Geometry check sheet. Reference: the model listing, model coordinates, mm. Face numbers are marked on the shaded views. A direction names the side the tool comes from. Round coordinates to 2 decimals unless told otherwise and drop trailing zeros. Write each loop counter-clockwise with the first axis right and the second up, starting at its lowest first coordinate (ties: lowest second). Pieces come first, ordered by that corner, then holes. Notation, with made-up numbers: M 86.5,-38.75 L 96.5,-38.75 A14 ccw 96.5,-14.75 Z; hole C 67.5,80.5 d7. An arc over 180 degrees is marked long. Use a Markdown table: item, result.
```python
from build123d import *

# Parameters (mm, degrees)
F1_DEPTH      = 12.7
F1_DEPTH_BACK = 12.7
F2_R          = 3.937
F3_DEPTH      = 25.401
F5_W          = 25.4239097328
F5_H          = 19.05
F6_DEPTH      = 20.9247035883
F6_DEPTH_BACK = 20.2536193136


with BuildPart() as f1:
    # F0 (on Front) → F1 (new body, two sides)
    with BuildSketch(Plane.XZ) as f1_sk:
        with BuildLine():
            Line((622.2402070197, 68.0433236969), (599.7125589726, 54.4963749958))
            ThreePointArc((599.7125589726, 54.4963749958), (596.4317742001, 46.7743526151), (602.7544880205, 41.259239895))
            Line((602.7544880205, 41.259239895), (604.0336175771, 41.259239895))
            Line((604.0336175771, 41.259239895), (628.785084933, 41.259239895))
            Line((628.785084933, 41.259239895), (644.685484933, 41.259239895))
            Line((644.685484933, 41.259239895), (644.685484933, 57.159639895))
            Line((644.685484933, 57.159639895), (641.485084933, 57.159639895))
            ThreePointArc((641.485084933, 57.159639895), (622.5332831727, 46.1050040009), (622.2402070197, 68.0433236969))
        make_face()
        with BuildLine():
            Line((604.0336175771, 41.259239895), (602.7544880205, 41.259239895))
            ThreePointArc((602.7544880205, 41.259239895), (603.3940527988, 41.2305528572), (604.0336175771, 41.259239895))
        make_face()
    extrude(amount=F1_DEPTH)
    extrude(f1_sk.sketch, amount=-F1_DEPTH_BACK)

    # F2 (on face) → F3 (cut, through all)
    with BuildSketch(Plane(origin=(0, 12.7, 0), x_dir=(-1, 0, 0), z_dir=(0, 1, 0))):
        with Locations((-603.3940527988, 48.3743028572)):
            Circle(F2_R)
    extrude(amount=-F3_DEPTH, mode=Mode.SUBTRACT)

    # F5 (on face) → F6 (cut, two sides)
    with BuildSketch(Plane(origin=(49.5651934259, 0, -143.2513532049), x_dir=(0.9450305474, 0, 0.3269820552), z_dir=(0.3269820552, 0, -0.9450305474))) as f6_sk:
        with Locations((584.3355135098, 0)):
            Rectangle(F5_W, F5_H)
    extrude(amount=-F6_DEPTH, mode=Mode.SUBTRACT)
    extrude(f6_sk.sketch, amount=F6_DEPTH_BACK, mode=Mode.SUBTRACT)


solid = f1.part
```
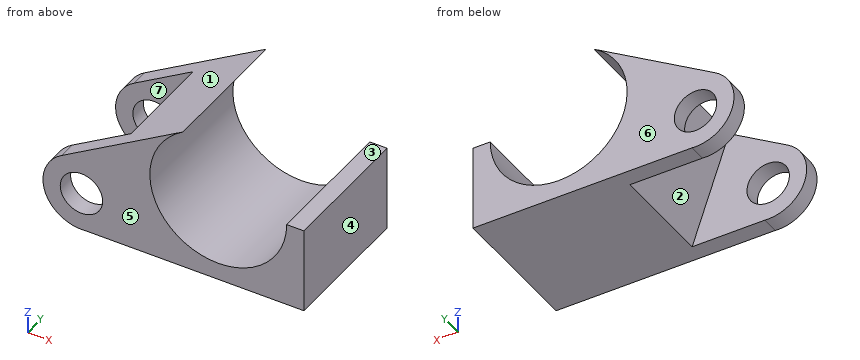
Item 1: Material ranges on line 1 along Y through (x, z) = (608.5, 57) (3 decimals); line 2 along X through (y, z) = (3, 56.25); line 3 along X through (y, z) = (7, 55.75), recorded low to high. Write a range as from..to.
Outcome:
| item | result |
|---|---|
| line 1 | y = -12.7..-9.525, 9.525..12.7 |
| line 2 | x = 612.31..616.12, 641.45..644.69 |
| line 3 | x = 612.49..616.16, 641.41..644.69 |
Item 2: Cross-section at A-A, the plane z = 55. Record the cut outline in (x, y) (3 decimals).
Outcome:
| item | result |
|---|---|
| outline | M 600.55,-12.7 L 616.27,-12.7 L 616.27,12.7 L 600.55,12.7 L 600.55,9.525 L 612.746,9.525 L 612.746,-9.525 L 600.55,-9.525 Z; M 641.3,-12.7 L 644.685,-12.7 L 644.685,12.7 L 641.3,12.7 Z |
Item 3: Cross-section at C-C, the plane y = 6.25. Record the cut outline in (x, z), and give its area (3 significant figures).
Outcome:
| item | result |
|---|---|
| outline | M 610.65,61.07 L 617.5,41.26 L 644.69,41.26 L 644.69,57.16 L 641.49,57.16 A12.7 cw long 622.24,68.04 Z |
| area | 258 mm2 |
Item 4: Go/stop test with flat-tipped pins: pin 1 (6 mm diameter, centred on x = 611, y = -6.5, fed in from +Z); pin 2 (4 mm diameter, centred on x = 637, y = -2.5, fed in from +Z); pin 3 (8 mm diameter, centred on y = 4.5, z = 44, fed in from -X); pin 4 (8 mm diameter, centred on x = 620.5, z = 49, fed in from +Y). Record where each tip stops, or that it passes through.
Outcome:
| item | result |
|---|---|
| pin 1 | stops at z = 63.09 |
| pin 2 | stops at z = 49.61 |
| pin 3 | stops at x = 615.17 |
| pin 4 | stops at y = 12.7 |
Item 5: Mould release check, pull along Y, two halves, no side actions. Record for the marked faces 4, 5, 6 and 7: +Y half, -Y half, draft (parallel to the pull), parting line (faces both ways), or undercut.
Outcome:
| item | result |
|---|---|
| face 4 | draft |
| face 5 | -Y half |
| face 6 | +Y half |
| face 7 | undercut |
Item 6: Access from +Z, -Z, +X, -X, +Y, -Y to the whole of each face (thin tool, end or side, straight path). Record for the marked faces 1, 2 and 3.
Outcome:
| item | result |
|---|---|
| face 1 | +Z, -X, +Y, -Y |
| face 2 | -Z, -X |
| face 3 | +Z, +X, +Y, -Y |
Item 7: Cross-section at D-D, the plane z = 59. Record the cut outline in (x, y) (3 decimals).
Outcome:
| item | result |
|---|---|
| outline | M 607.202,-12.7 L 616.219,-12.7 L 616.219,12.7 L 607.202,12.7 L 607.202,9.525 L 611.362,9.525 L 611.362,-9.525 L 607.202,-9.525 Z |
